For this review, use the dimensioned drawing (mm, ordinates from the lowest corner) and the shaded views. A direction names the side the tool comes from. Round coordinates to 2 decimals unless told otherwise and drop trailing zeros. Loops run counter-clockwise (first coordinate to the right, second up) from the corner with the lowest first, then second, coordinate; pieces in that order, holes last. Notation, with made-up numbers: M 86.5,-21.5 L 138.5,-21.5 A24 ccw 138.5,-11.5 Z; hole C -24.5,37 d7. An arc over 180 degrees is marked long. Answer as a JSON object with one key per item and string values. Group by question number.
Item 1: Consider section D-D (x = 57.5). Give the boundary of the cut face in (y, z).
Item 2: To check wall thickness, follow line 1 (Y direction, x = 19.5, z = 30.5); line 2 (X direction, y = 12.75, z = 27.5); line 3 (Z direction, x = 6, y = 10.5). State the ranges of each line that lie inside material, in increasing order.
Item 3: Insertion check: P1, Ø1, axis at x = 70, z = 21.5, coming from the -Y side; P2, Ø1.5, axis at x = 39, y = 12.5, coming from the -Z side; P3, Ø0.8, axis at y = 3.5, z = 2.5, coming from the -X side. Each pin has a flat end and moves straight along its axis. Give the tip position at first contact, or say it passes through.
Item 4: Consider section A-A (x = 40). Give the boundary of the cut face in (y, z).
Item 5: Tool access review of the marked faces 1, 2, 3, 4 and 5: name each direction out of +Z, -Z, +X, -X, +Y, -Y from which nothing blocks a thin tool from reaching the whole face with its end or side.
Item 6: Consider section B-B (z = 24). Give the boundary of the cut face in (x, y), and give its area (3 significant figures).
Item 7: Consider section C-C (y = 11.75). Give the boundary of the cut face in (x, z).
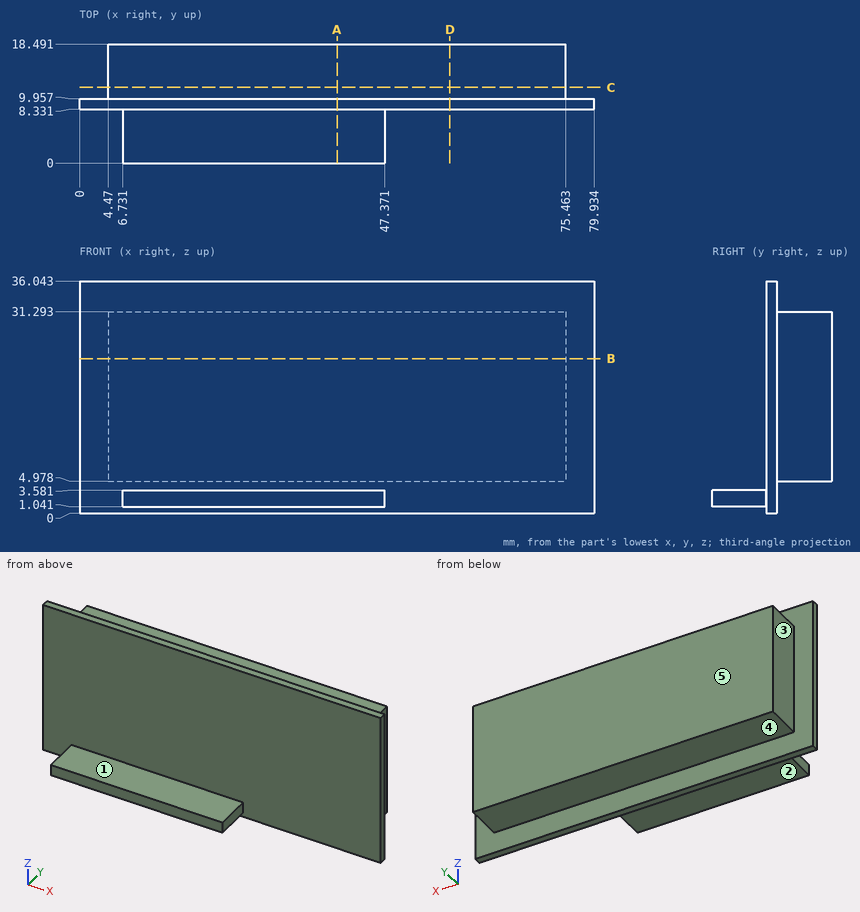
Geometry results:
{
 "1": {"outline": "M 8.33,0 L 9.96,0 L 9.96,4.98 L 18.49,4.98 L 18.49,31.29 L 9.96,31.29 L 9.96,36.04 L 8.33,36.04 Z"},
 "2": {"line 1": "y = 8.33 to 18.49", "line 2": "x = 4.47 to 75.46", "line 3": "z = 4.98 to 31.29"},
 "3": {"P1": "stops at y = 8.33", "P2": "stops at z = 4.98", "P3": "stops at x = 6.73"},
 "4": {"outline": "M 0,1.04 L 8.33,1.04 L 8.33,0 L 9.96,0 L 9.96,4.98 L 18.49,4.98 L 18.49,31.29 L 9.96,31.29 L 9.96,36.04 L 8.33,36.04 L 8.33,3.58 L 0,3.58 Z"},
 "5": {"face 1": "+Z, +X, -X, -Y", "face 2": "-Z, +X, -X, -Y", "face 3": "+Z, -Z, -X, +Y", "face 4": "-Z, +X, -X, +Y", "face 5": "+Z, -Z, +X, -X, +Y"},
 "6": {"outline": "M 0,8.33 L 79.93,8.33 L 79.93,9.96 L 75.46,9.96 L 75.46,18.49 L 4.47,18.49 L 4.47,9.96 L 0,9.96 Z", "area": "736 mm^2"},
 "7": {"outline": "M 4.47,4.98 L 75.46,4.98 L 75.46,31.29 L 4.47,31.29 Z"}
}
